Part print with two shaded views. Sizes in mm from the minimum x, y, z corner. A direction names the side the tool comes from. Round coordinates to 2 decimals unless told otherwise and drop trailing zeros. Order: outer loops, then holes, each group sorted by start corner. A loop starts at its lowest first (then second) coordinate and runs counter-clockwise, first axis right, second up. Notation, with made-up numbers: M 70.25,30 L 109.25,30 A27 ccw 109.25,62 Z; hole C -23,-36.75 d2. An arc over 180 degrees is marked long. Answer as a JSON object with one key per item and string values.
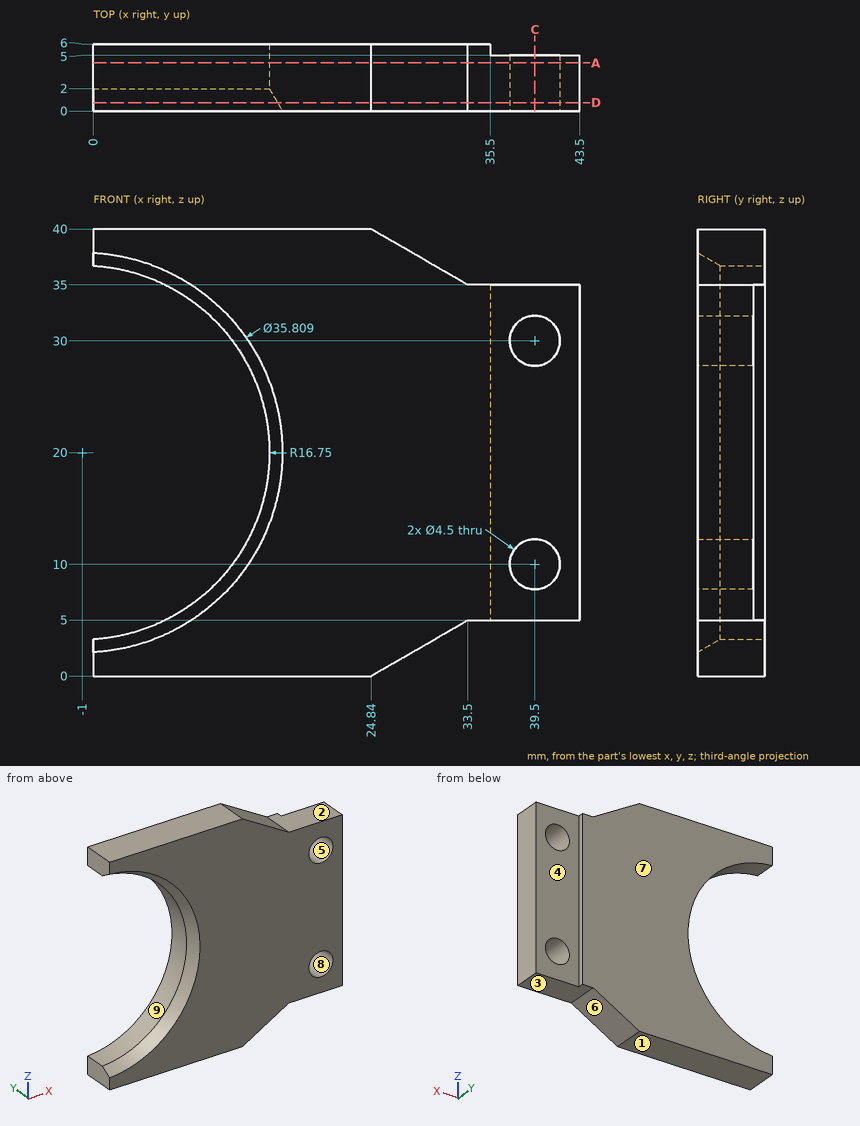
Item 1: Drop flat-ended pins along their axis: pin 1 Ø6 at (x, z) = (39.5, 30) entering from +Y; pin 2 Ø7 at (x, z) = (39.5, 10) entering from -Y; pin 3 Ø1.8 at (x, y) = (39, 2.5) entering from +Z; pin 4 Ø1.8 at (x, y) = (40, 1.5) entering from -Z. Give the stop position or say it passes through.
Worked answers:
{"pin 1": "stops at y = 5", "pin 2": "stops at y = 0", "pin 3": "stops at z = 35", "pin 4": "stops at z = 5"}
Item 2: 3-axis set-ups, long thin cutter, end or side, ignore diameter. For the marked faces 1, 2, 3, 4 and 5: which of +Z, -Z, +X, -X, +Y, -Y reach the whole face in a straight line?
Worked answers:
{"face 1": "-Z, +X, -X, +Y, -Y", "face 2": "+Z, +X, +Y, -Y", "face 3": "-Z, +X, +Y, -Y", "face 4": "+Z, -Z, +X, +Y", "face 5": "+Y, -Y"}
Item 3: Saw through at D-D on y = 0.75. List the corners of the cut face in (x, z), and give its area (3 significant figures).
Worked answers:
{"outline": "M 0,0 L 24.84,0 L 33.5,5 L 43.5,5 L 43.5,35 L 33.5,35 L 24.84,40 L 0,40 L 0,37.44 A17.47 cw 0,2.56 Z; hole C 39.5,10 d4.5; hole C 39.5,30 d4.5", "area": "1,120 mm2"}
Item 4: Two-plate mould, pull along Z, no slides. Class the marked faces 6, 7, 8 and 9: released by +Z, released by -Z, zero draft, split by the parting line, or undercut.
Worked answers:
{"face 6": "released by -Z", "face 7": "zero draft", "face 8": "undercut", "face 9": "undercut"}
Item 5: Saw through at C-C on x = 39.5. List the corners of the cut face in (y, z), and give its area (3 significant figures).
Worked answers:
{"outline": "M 0,5 L 5,5 L 5,7.75 L 0,7.75 Z; M 0,12.25 L 5,12.25 L 5,27.75 L 0,27.75 Z; M 0,32.25 L 5,32.25 L 5,35 L 0,35 Z", "area": "105 mm2"}
Item 6: Wall check: line 1 along Z through (x, y) = (39.5, 2.5); line 2 along Z through (x, y) = (38, 2) (1 decimal); line 3 along Y through (x, z) = (37, 26). Give the ranges that are in metal, low to high. Write a range as [from, to].
Worked answers:
{"line 1": "z = [5, 7.75], [12.25, 27.75], [32.25, 35]", "line 2": "z = [5, 8.3], [11.7, 28.3], [31.7, 35]", "line 3": "y = [0, 5]"}
Item 7: Saw through at A-A on y = 4.3. List the corners of the cut face in (x, z).
Worked answers:
{"outline": "M 0,0 L 24.84,0 L 33.5,5 L 43.5,5 L 43.5,35 L 33.5,35 L 24.84,40 L 0,40 L 0,36.72 A16.75 cw 0,3.28 Z; hole C 39.5,10 d4.5; hole C 39.5,30 d4.5"}
